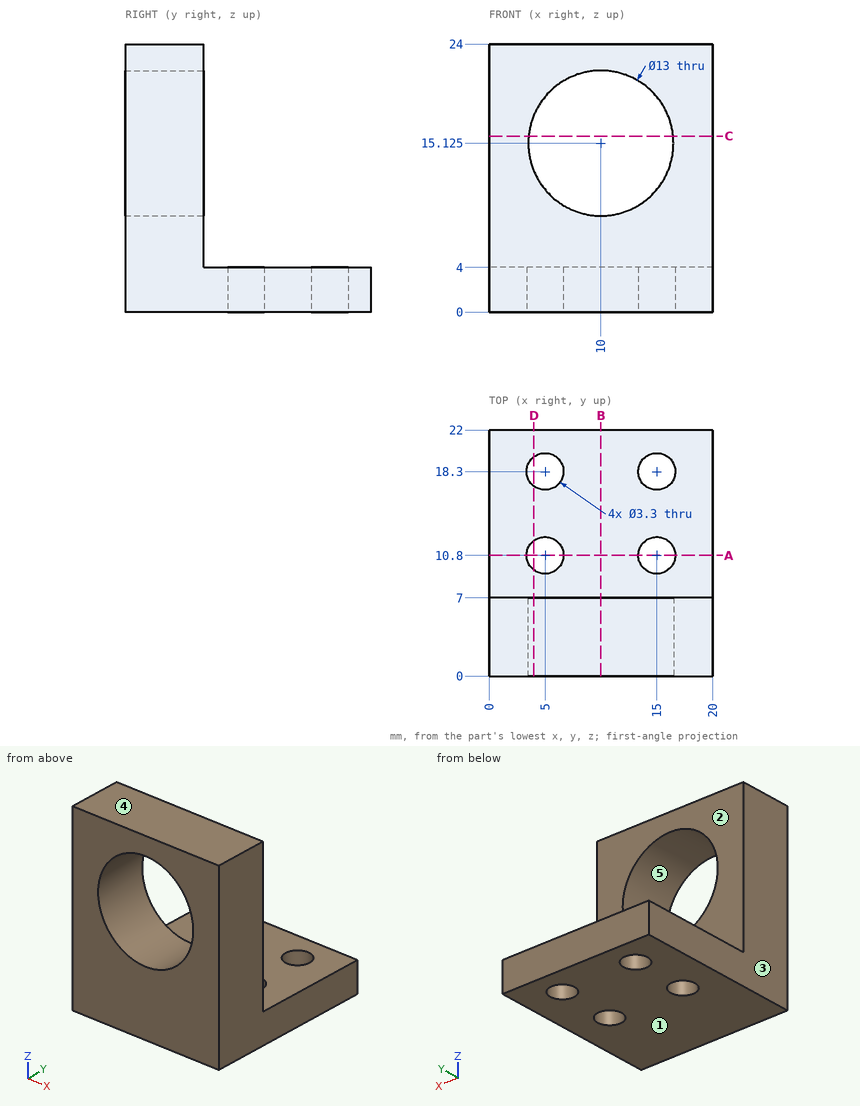
Verification items for this drawing (mm, ordinates from the low corner). A direction names the side the tool comes from. Round coordinates to 2 decimals unless told otherwise and drop trailing zeros. Loops run counter-clockwise (first coordinate to the right, second up) from the corner with the lowest first, then second, coordinate; pieces in that order, holes last. Notation, with made-up numbers: (35, 67) -> (64, 67) arc R19 ccw to (64, 87) -> close; hole circle Ø11 at (82.5, -27). An arc over 180 degrees is marked (long way). Write item = value, one per line. Start each with the question number.
1) Sectioned sample at D-D, the plane x = 4. Record the cut outline in (y, z) (3 decimals).
2) Set-up check for the marked faces 1 and 2: record each of +Z, -Z, +X, -X, +Y, -Y from which the full face is reachable in a straight line by a thin tool's end or side.
3) Sectioned sample at B-B, the plane x = 10. Record the cut outline in (y, z) (3 decimals), plus the area to 3 significant figures.
4) Sectioned sample at C-C, the plane z = 15.75. Record the cut outline in (x, y).
5) Sectioned sample at A-A, the plane y = 10.8. Record the cut outline in (x, z).
6) Gauge pin test, flat ends, axial feed: pin 1 Ø12 at (y, z) = (3, 9) entering from -X; pin 2 Ø6 at (x, y) = (12, 17) entering from +Z; pin 3 Ø1 at (x, z) = (2.5, 9) entering from +Y. Record the tip position at first contact, or that the pin passes through.
7) Thickness scan on probe 1 along Y at (x, z) = (5, 1.4); probe 2 along X at (y, z) = (18.3, 2.7); probe 3 along X at (y, z) = (19, 3.25). Record the ranges inside material, lowest first.
8) Release check for a two-part mould opening along X. For the marked faces 3, 4 and 5 record: released by +X, released by -X, zero draft, split by the parting line, or undercut.
Results are:
q1.outline = (0, 0) -> (9.488, 0) -> (9.488, 4) -> (7, 4) -> (7, 12.625) -> (0, 12.625) -> close; (0, 17.625) -> (7, 17.625) -> (7, 24) -> (0, 24) -> close; (12.112, 0) -> (16.988, 0) -> (16.988, 4) -> (12.112, 4) -> close; (19.612, 0) -> (22, 0) -> (22, 4) -> (19.612, 4) -> close
q2.face_1 = -Z, +X, -X, +Y, -Y
q2.face_2 = +Z, +X, -X, +Y
q3.outline = (0, 0) -> (22, 0) -> (22, 4) -> (7, 4) -> (7, 8.625) -> (0, 8.625) -> close; (0, 21.625) -> (7, 21.625) -> (7, 24) -> (0, 24) -> close
q3.area = 137 mm^2
q4.outline = (0, 0) -> (3.53, 0) -> (3.53, 7) -> (0, 7) -> close; (16.47, 0) -> (20, 0) -> (20, 7) -> (16.47, 7) -> close
q5.outline = (0, 0) -> (3.35, 0) -> (3.35, 4) -> (0, 4) -> close; (6.65, 0) -> (13.35, 0) -> (13.35, 4) -> (6.65, 4) -> close; (16.65, 0) -> (20, 0) -> (20, 4) -> (16.65, 4) -> close
q6.pin_1 = 0
q6.pin_2 = 4
q6.pin_3 = 7
q7.probe_1 = 0 to 9.15, 12.45 to 16.65, 19.95 to 22
q7.probe_2 = 0 to 3.35, 6.65 to 13.35, 16.65 to 20
q7.probe_3 = 0 to 3.51, 6.49 to 13.51, 16.49 to 20
q8.face_3 = released by -X
q8.face_4 = zero draft
q8.face_5 = undercut
